The model under review builds one solid part; all positions refer to its coordinate system, in mm. A direction names the side the tool comes from. Round coordinates to 2 decimals unless told otherwise and drop trailing zeros. Order: outer loops, then holes, each group sorted by start corner. A loop starts at its lowest first (then second) coordinate and runs counter-clockwise, first axis right, second up. Notation, with made-up numbers: (52.5, 57.25) -> (87.5, 57.25) arc R21 cw to (87.5, 74.25) -> close; hole circle Ø5 at (88, 59). An arc over 180 degrees is marked (long way). Use a Markdown table: item, result. Add a question column.
```python
from build123d import *

# Parameters (mm, degrees)
EXTRUDE1_DEPTH = 12.7


with BuildPart() as part:
    # Sketch1 → Extrude1 (new, symmetric)
    with BuildSketch(Plane.XY):
        with BuildLine():
            Line((-105.256684146, 30.159371772), (-35.906883315, 67.209640161))
            ThreePointArc((-35.906883315, 67.209640161), (-31.500545183, 69.384116721), (-26.963222432, 71.270082335))
            ThreePointArc((-26.963222432, 71.270082335), (64.384642533, 40.75607692), (52.880823594, -54.864))
            ThreePointArc((52.880823594, -54.864), (38.665343582, -64.081234212), (22.033676498, -67.31))
            Line((22.033676498, -67.31), (-101.6, -67.31))
            ThreePointArc((-101.6, -67.31), (-135.901703173, -49.47989326), (-141.016910096, -11.160783079))
            ThreePointArc((-141.016910096, -11.160783079), (-126.968198666, 12.815152805), (-105.256684146, 30.159371772))
        make_face()
        with BuildLine():
            Line((19.364916731, 5), (25, 5))
            Line((25, 5), (25, -5))
            Line((25, -5), (19.364916731, -5))
            ThreePointArc((19.364916731, -5), (-20, 0), (19.364916731, 5))
        make_face(mode=Mode.SUBTRACT)
    extrude(amount=EXTRUDE1_DEPTH, both=True)


solid = part.part
```
Q1. To check wall thickness, follow line 1 along Y through (x, z) = (0, 6.5); line 2 along X through (y, z) = (0.5, 9.25); line 3 along X through (y, z) = (0, -1.25). State the ranges of each line that lie inside material, in increasing order.
Q2. Add section C-C, the plane y = 0. Give the boundary of the cut face in (x, z), then the cut area to 3 significant figures.
Q3. For pin 1 (6 mm diameter, centred on x = 23, z = -1, fed in from -Y); pin 2 (6 mm diameter, centred on y = -51, z = -4.5, fed in from +X); pin 3 (6 mm diameter, centred on x = 22, z = 1.5, fed in from +Y); pin 4 (1 mm diameter, centred on y = -23.5, z = -7.5, fed in from +X), all flat-tipped, find the tip position at first contact; note any pin that passes through.
Q4. For faces 1 (the face through (-39, -67.31, 0)), 2 (the face through (22, -5, 0)), list the 3-axis set-ups (+Z, -Z, +X, -X, +Y, -Y) from which the entire face can be reached by the end or side of a thin tool; tool diameter is ignored.
Q5. Add section A-A, the plane x = 0. Give the boundary of the cut face in (y, z), then the cut area to 3 significant figures.
Q6. Add section D-D, the plane x = 38. Give the boundary of the cut face in (y, z).
Q7. Draft analysis for pull direction X (two halves, no side actions). For faces 3 (the face through (38.89, -63.99, 0.18)), 4 (the face through (-19.984, -0.809, 0.178)), 5 (the face through (-71.067, 48.425, 0.178)), 6 (the face through (22, 5, 0)), state which applies: released by +X, released by -X, zero draft, split by the parting line, or undercut.
Q8. Add section B-B, the plane z = -0.25. Give the boundary of the cut face in (x, y).
Return value:
| question | item | result |
|---|---|---|
| 1 | line 1 | -67.31 to -20, 20 to 76.2 |
| 1 | line 2 | -135.66 to -19.99, 25 to 76.2 |
| 1 | line 3 | -135.94 to -20, 25 to 76.2 |
| 2 | outline | (-135.94, -12.7) -> (-20, -12.7) -> (-20, 12.7) -> (-135.94, 12.7) -> close; (25, -12.7) -> (76.2, -12.7) -> (76.2, 12.7) -> (25, 12.7) -> close |
| 2 | area | 4,250 mm² |
| 3 | pin 1 | y = -67.31 |
| 3 | pin 2 | x = 59.18 |
| 3 | pin 3 | y = 73.79 |
| 3 | pin 4 | x = 72.65 |
| 4 | face 1 | +Z, -Z, +X, -X, -Y |
| 4 | face 2 | +Z, -Z |
| 5 | outline | (-67.31, -12.7) -> (-20, -12.7) -> (-20, 12.7) -> (-67.31, 12.7) -> close; (20, -12.7) -> (76.2, -12.7) -> (76.2, 12.7) -> (20, 12.7) -> close |
| 5 | area | 2,630 mm² |
| 6 | outline | (-64.34, -12.7) -> (66.05, -12.7) -> (66.05, 12.7) -> (-64.34, 12.7) -> close |
| 7 | face 3 | released by +X |
| 7 | face 4 | undercut |
| 7 | face 5 | released by -X |
| 7 | face 6 | undercut |
| 8 | outline | (-141.02, -11.16) arc R41.91 ccw to (-101.6, -67.31) -> (22.03, -67.31) arc R44.45 ccw to (52.88, -54.86) arc R76.2 ccw to (-35.91, 67.21) -> (-105.26, 30.16) arc R76.2 ccw to start; hole (19.36, -5) -> (25, -5) -> (25, 5) -> (19.36, 5) arc R20 ccw (long way) to start |
